Study the drawing (mm; zero at the part's minimum x, y, z) and answer. Round coordinates to 2 decimals unless told otherwise and drop trailing zeros. Write each loop counter-clockwise with the first axis right and the second up, starting at its lowest first coordinate (ties: lowest second). Pieces come first, ordered by that corner, then holes. Notation, with made-up numbers: M 13,1.5 L 42,1.5 A22 ccw 42,22.5 Z; hole C -37.5,59.25 d2. An arc over 180 degrees is marked long. Put each result on its own line as item: value. Start each with the question number.
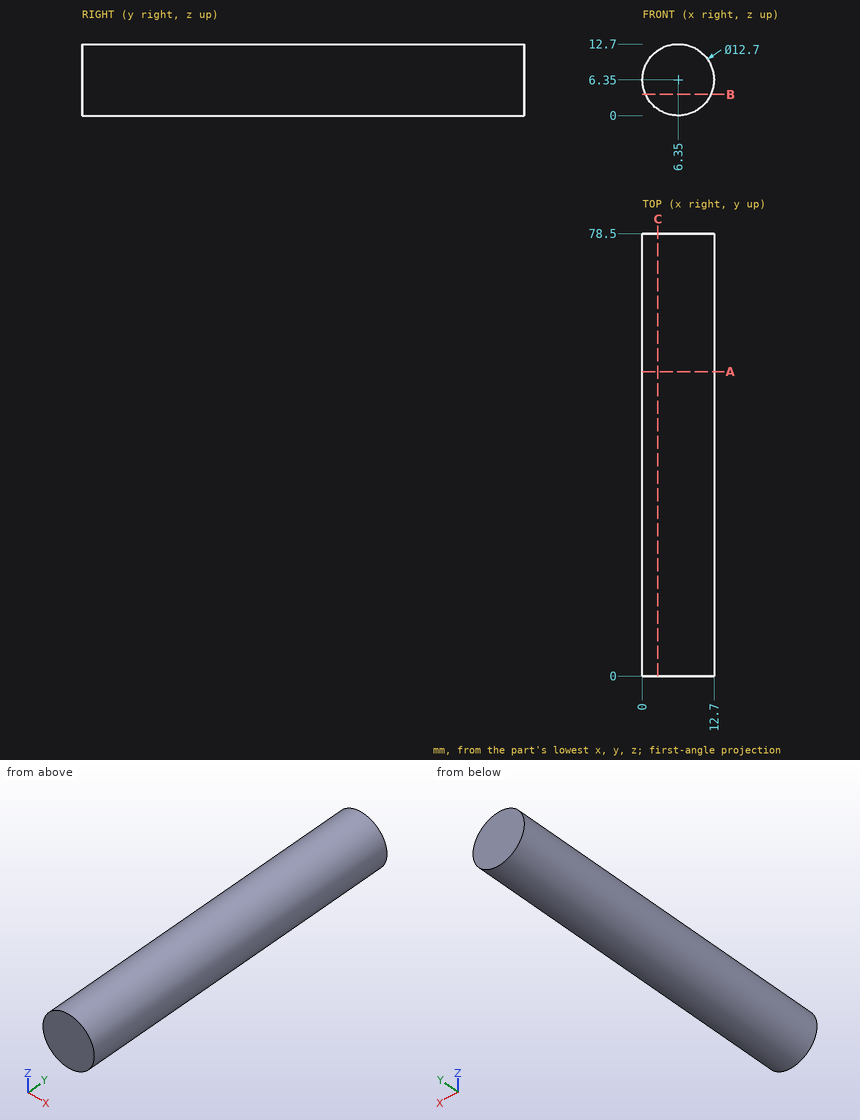
Item 1: Section B-B (z = 3.75) is taken. Give the vertices of the cut face in (x, y), and give its area (3 significant figures).
Item 2: Flat-ended cylindrical pins translate along their axes: pin 1 (4 mm diameter, centred on x = 3.5, z = 5.5, fed in from -Y); pin 2 (3 mm diameter, centred on x = 10, y = 34.5, fed in from -Z); pin 3 (2 mm diameter, centred on x = 1.5, y = 63.5, fed in from -Z); pin 4 (3 mm diameter, centred on y = 51, z = 3.5, fed in from -X). Find the tip coordinate at first contact, or state that the pin passes through.
Item 3: Consider line 1 along X through (y, z) = (5.5, 6.75); line 2 along X through (y, z) = (34, 5.5); line 3 along Z through (x, y) = (8.75, 37.5). Determine where each line is inside the solid, lowest interval first. Write a range as [from, to].
Item 4: Section A-A (y = 54) is taken. Give the vertices of the cut face in (x, z), and give its area (3 significant figures).
Item 5: Section C-C (x = 2.75) is taken. Give the vertices of the cut face in (y, z).
Output values:
1. outline: M 0.56,0 L 12.14,0 L 12.14,78.5 L 0.56,78.5 Z
1. area: 910 mm^2
2. pin 1: stops at y = 0
2. pin 2: stops at z = 0.38
2. pin 3: stops at z = 1.3
2. pin 4: stops at x = 0.15
3. line 1: x = [0.01, 12.69]
3. line 2: x = [0.06, 12.64]
3. line 3: z = [0.47, 12.23]
4. outline: C 6.35,6.35 d12.7
4. area: 127 mm^2
5. outline: M 0,1.12 L 78.5,1.12 L 78.5,11.58 L 0,11.58 Z
